Here's how the part is built. I have some questions about the finished solid (model axes, mm). A direction names the side the tool comes from. Round coordinates to 2 decimals unless told otherwise and drop trailing zeros. Write each loop counter-clockwise with the first axis right and the second up, starting at its lowest first coordinate (ties: lowest second). Pieces come first, ordered by that corner, then holes. Notation, with made-up numbers: M 46,24.5 L 66,24.5 A12 cw 66,33.5 Z; hole C 66.5,43 d3. An arc over 180 degrees is marked long. Use a Markdown table: item, result. Add a question column.
```python
from build123d import *

# Parameters (mm, degrees)
BOSS_EXTRU_1_DEPTH      = 10
BOSS_EXTRU_2_DEPTH      = 10
ENL_V_MAT_EXTRU_1_REACH = 37.775
ENL_V_MAT_EXTRU_2_REACH = 34.103
ESQUISSE4_R             = 2.75
ENL_V_MAT_EXTRU_3_REACH = 37.12
ESQUISSE5_R             = 2.1
CHANFREIN1_SIZE         = 10
ENL_V_MAT_EXTRU_4_REACH = 42.247
ENL_V_MAT_EXTRU_5_REACH = 47.329
ESQUISSE7_R             = 1.25


with BuildPart() as part:
    # Esquisse1 → Boss.-Extru.1 (new body)
    with BuildSketch(Plane.XY):
        Polygon((0, 0), (29.25, 0), (29.25, 10), (10, 10), (10, 22), (0, 22), align=None)
    extrude(amount=BOSS_EXTRU_1_DEPTH)

    # Esquisse2 → Boss.-Extru.2 (add)
    with BuildSketch(Plane(origin=(0, 10, 0), x_dir=(1, 0, 0), z_dir=(0, 1, 0))):
        Polygon((29.25, 0), (26.29798098, 16.741731801), (21.373942215, 15.873490913), (24.172866941, 0), align=None)
        Polygon((16.557167351, 0), (13.987884067, 14.57112958), (9.063845302, 13.702888692), (11.480034292, 0), align=None)
    extrude(amount=-BOSS_EXTRU_2_DEPTH)

    # Esquisse3 → Enlèv. mat.-Extru.1 (cut, up to next)
    with BuildSketch(Plane(origin=(0, 10, 0), x_dir=(1, 0, 0), z_dir=(0, 1, 0)), mode=Mode.PRIVATE) as enl_v_mat_extru_1_sk1:
        Polygon((16.557167351, 0), (16.817639618, -1.47721163), (24.203697766, -0.174850297), (24.172866941, 0), align=None)
    enl_v_mat_extru_1_tool1 = extrude(enl_v_mat_extru_1_sk1.sketch, amount=-ENL_V_MAT_EXTRU_1_REACH, mode=Mode.PRIVATE) & part.part
    add(enl_v_mat_extru_1_tool1.solids().sort_by_distance((19.452321, 10, 0.498572))[0], mode=Mode.SUBTRACT)

    # Esquisse4 → Enlèv. mat.-Extru.2 (cut, up to next)
    with BuildSketch(Plane(origin=(11.133868901, 0, -1.963201487), x_dir=(0.1736481776669311, 0, 0.9848077530122079), z_dir=(-0.9848077530122079, 0, 0.1736481776669311)), mode=Mode.PRIVATE) as enl_v_mat_extru_2_sk1:
        with Locations((-4.006512966, 6)):
            Circle(ESQUISSE4_R)
    enl_v_mat_extru_2_tool1 = extrude(enl_v_mat_extru_2_sk1.sketch, amount=-ENL_V_MAT_EXTRU_2_REACH, mode=Mode.PRIVATE) & part.part
    add(enl_v_mat_extru_2_tool1.solids().sort_by_distance((10.438145, 6, -5.908847))[0], mode=Mode.SUBTRACT)

    # Esquisse5 → Enlèv. mat.-Extru.3 (cut, up to next)
    with BuildSketch(Plane(origin=(23.443965814, 0, -4.133803708), x_dir=(0.1736481776669306, 0, 0.9848077530122081), z_dir=(-0.9848077530122081, 0, 0.1736481776669306)), mode=Mode.PRIVATE) as enl_v_mat_extru_3_sk1:
        with Locations((-4.006512966, 6)):
            Circle(ESQUISSE5_R)
    enl_v_mat_extru_3_tool1 = extrude(enl_v_mat_extru_3_sk1.sketch, amount=-ENL_V_MAT_EXTRU_3_REACH, mode=Mode.PRIVATE) & part.part
    add(enl_v_mat_extru_3_tool1.solids().sort_by_distance((22.748242, 6, -8.079449))[0], mode=Mode.SUBTRACT)

    # Chanfrein1
    chanfrein1_edges = [part.edges().sort_by_distance(p)[0] for p in [
        (29.25, 5, 10),
    ]]
    chamfer(chanfrein1_edges, length=CHANFREIN1_SIZE - 0.0001)  # a hair under: the kernel refuses the full size

    # Esquisse6 → Enlèv. mat.-Extru.4 (cut, up to next)
    with BuildSketch(Plane(origin=(0, 22, 0), x_dir=(1, 0, 0), z_dir=(0, 1, 0)), mode=Mode.PRIVATE) as enl_v_mat_extru_4_sk1:
        Polygon((0, 0), (11.480034292, 0), (0, -2.024239785), align=None)
    enl_v_mat_extru_4_tool1 = extrude(enl_v_mat_extru_4_sk1.sketch, amount=-ENL_V_MAT_EXTRU_4_REACH, mode=Mode.PRIVATE) & part.part
    add(enl_v_mat_extru_4_tool1.solids().sort_by_distance((3.826678, 22, 0.674747))[0], mode=Mode.SUBTRACT)

    # Enlèv. mat.-Extru.5: up to this plane
    enl_v_mat_extru_5_end = Plane(origin=(11.480034292, -0.001, 0), z_dir=(0.1736481776669316, 0, 0.9848077530122079))
    # Esquisse7 → Enlèv. mat.-Extru.5 (cut, up to the surface)
    with BuildSketch(Plane.XY.offset(10), mode=Mode.PRIVATE) as enl_v_mat_extru_5_sk1:
        with Locations((5.19, 17)):
            Circle(ESQUISSE7_R)
    enl_v_mat_extru_5_tool1 = split(extrude(enl_v_mat_extru_5_sk1.sketch, amount=-ENL_V_MAT_EXTRU_5_REACH, mode=Mode.PRIVATE), bisect_by=enl_v_mat_extru_5_end, keep=Keep.BOTH, mode=Mode.PRIVATE)
    add(enl_v_mat_extru_5_tool1.solids().sort_by_distance((5.19, 17, 10))[0], mode=Mode.SUBTRACT)
    # Esquisse7 → Enlèv. mat.-Extru.5 (cut, up to the surface)
    with BuildSketch(Plane.XY.offset(10), mode=Mode.PRIVATE) as enl_v_mat_extru_5_sk2:
        with Locations((5.19, 9.22)):
            Circle(ESQUISSE7_R)
    enl_v_mat_extru_5_tool2 = split(extrude(enl_v_mat_extru_5_sk2.sketch, amount=-ENL_V_MAT_EXTRU_5_REACH, mode=Mode.PRIVATE), bisect_by=enl_v_mat_extru_5_end, keep=Keep.BOTH, mode=Mode.PRIVATE)
    add(enl_v_mat_extru_5_tool2.solids().sort_by_distance((5.19, 9.22, 10))[0], mode=Mode.SUBTRACT)


solid = part.part
```
Item 1: Imagine slicing it at D-D on z = 3.5. List the corners of the cut face in (x, y) for me.
Item 2: Imagine slicing it at C-C on x = 21.75. List the corners of the cut face in (y, z) for me.
Item 3: Imagine slicing it at B-B on y = 17. List the corners of the cut face in (x, z) for me, plus the area to 3 significant figures.
Item 4: I need wall thicknesses on probe 1 along Y at (x, z) = (5.19, 6.75); probe 2 along Y at (x, z) = (5.5, 6.75); probe 3 along X at (y, z) = (17, 3.5). Which ranges of each line are inside material? Lowest first, please. Write a range as from..to.
Item 5: For pin 1 Ø8 at (x, y) = (7.5, 6.5) entering from -Z; pin 2 Ø10.5 at (y, z) = (16.5, 4.5) entering from +X; pin 3 Ø6 at (x, z) = (23, 1) entering from +Y, each with a flat end and sliding along its axis, tell me the tip position at first contact or that it passes through.
Item 6: On a 3-axis mill with a long thin cutter (end or side, diameter ignored), from which of +Z, -Z, +X, -X, +Y, -Y can I reach the whole of each face in a straight line? I mean faces 1 (the face through (9.987, 3.959, -8.47)), 2 (the face through (10, 16, 5)), 3 (the face through (28.123, 5.07, -6.393)), 4 (the face through (20.459, 5.07, 0.835)). Say none if no direction works.
Item 7: If we mould it in two halves opening along Z, with no side actions, what happens to faces 5 (the face through (7, 9, 10)), 6 (the face through (15, 10, -1)), 7 (the face through (25.13, 8.08, -8.78))? For each: +Z half, -Z half, draft (parallel to the pull), parting line (faces both ways), or undercut.
The answers:
| question | item | result |
|---|---|---|
| 1 | outline | M 0,0 L 25.75,0 L 25.75,10 L 10,10 L 10,22 L 0,22 Z; hole C 5.19,9.22 d2.5; hole C 5.19,17 d2.5 |
| 2 | outline | M 0,-15.94 L 10,-15.94 L 10,-13.74 L 0,-13.74 Z; M 0,0.61 L 10,0.61 L 10,7.5 L 0,7.5 Z |
| 3 | outline | M 0,2.02 L 3.94,1.33 L 3.94,10 L 0,10 Z; M 6.44,0.89 L 10,0.26 L 10,10 L 6.44,10 Z |
| 3 | area | 66.3 mm² |
| 4 | probe 1 | 0..7.97, 10.47..15.75, 18.25..22 |
| 4 | probe 2 | 0..8.01, 10.43..15.79, 18.21..22 |
| 4 | probe 3 | 0..3.94, 6.44..10 |
| 5 | pin 1 | z = -14.13 |
| 5 | pin 2 | x = 10 |
| 5 | pin 3 | y = 10 |
| 6 | face 1 | -X, +Y, -Y |
| 6 | face 2 | +Z, -Z, +X, +Y |
| 6 | face 3 | -Z, +X, +Y, -Y |
| 6 | face 4 | +Y, -Y |
| 7 | face 5 | +Z half |
| 7 | face 6 | draft |
| 7 | face 7 | undercut |
